Read the model definition and answer for the solid it produces. Units are mm, in the model's axes. Coordinates: 2 decimals unless noted, no trailing zeros. Write each loop counter-clockwise with the first axis right and the second up, starting at its lowest first coordinate (ties: lowest second). Pieces come first, ordered by that corner, then holes. Notation, with made-up numbers: (-16.5, 59.5) -> (25.5, 59.5) arc R16 cw to (25.5, 90.5) -> close; hole circle Ø10 at (-24, 18.25). An arc over 180 degrees is marked (long way). One line per item, written item: value. Start each with the question number.
1. Find section C-C, the plane x = 1. Write down the section's boundary in (y, z).
2. Consider line 1 along X through (y, z) = (-28, 2.05); line 2 along Y through (x, z) = (97.5, 0.7); line 3 along Y through (x, z) = (89.5, 2.3). Determine where each line is inside the solid, lowest interval first.
3. Find section B-B, the plane z = 1.3. State how many separate pieces and enclosed holes the cut face has, and give its area (3 significant figures).
4. Given P1, Ø1.5, axis at y = -108.5, z = 1, coming from the +X side; P2, Ø4, axis at x = 113.5, y = -88, coming from the -Z side; P3, Ø1.5, axis at x = -151.5, z = 1.5, coming from the -Y side; P4, Ø0.9, axis at y = 108.5, z = 1, coming from the -X side, each flat-ended and moving along its own axis, determine where each tip first touches the part or whether it passes through.
5. Find section A-A, the plane y = -16. Write down the section's boundary in (x, z), and give its area (3 significant figures).
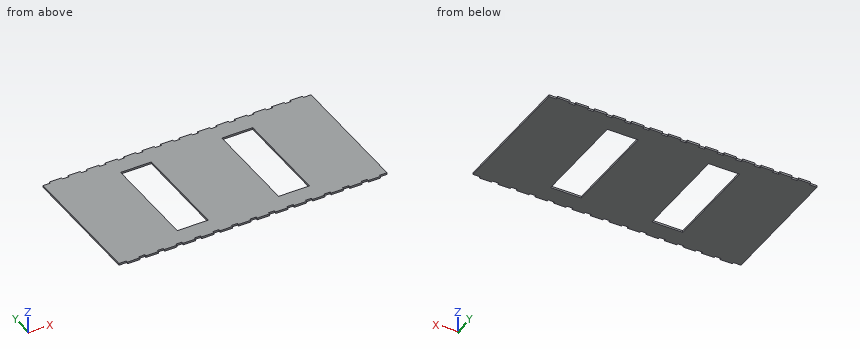
```python
from build123d import *

# Parameters (mm, degrees)
ESQUISSE1_W             = 434
ESQUISSE1_H             = 220
BOSS_EXTRU_1_DEPTH      = 3
ESQUISSE2_W             = 10
ESQUISSE2_H             = 3
ESQUISSE2_W_2           = 2
ENL_V_MAT_EXTRU_1_DEPTH = 3
ESQUISSE3_W             = 50
ESQUISSE3_H             = 160
ENL_V_MAT_EXTRU_2_DEPTH = 3


with BuildPart() as part:
    # Esquisse1 → Boss.-Extru.1 (new body)
    with BuildSketch(Plane.XY):
        Rectangle(ESQUISSE1_W, ESQUISSE1_H)
    extrude(amount=BOSS_EXTRU_1_DEPTH)

    # Esquisse2 → Enlèv. mat.-Extru.1 (cut)
    with BuildSketch(Plane.XY.offset(3)):
        with Locations((-210, 108.5)):
            Rectangle(ESQUISSE2_W, ESQUISSE2_H)
        with Locations((-180, 108.5)):
            Rectangle(ESQUISSE2_W, ESQUISSE2_H)
        with Locations((-150, 108.5)):
            Rectangle(ESQUISSE2_W, ESQUISSE2_H)
        with Locations((-120, 108.5)):
            Rectangle(ESQUISSE2_W, ESQUISSE2_H)
        with Locations((-90, 108.5)):
            Rectangle(ESQUISSE2_W, ESQUISSE2_H)
        with Locations((-30, 108.5)):
            Rectangle(ESQUISSE2_W, ESQUISSE2_H)
        with Locations((30, 108.5)):
            Rectangle(ESQUISSE2_W, ESQUISSE2_H)
        with Locations((60, 108.5)):
            Rectangle(ESQUISSE2_W, ESQUISSE2_H)
        with Locations((90, 108.5)):
            Rectangle(ESQUISSE2_W, ESQUISSE2_H)
        with Locations((120, 108.5)):
            Rectangle(ESQUISSE2_W, ESQUISSE2_H)
        with Locations((150, 108.5)):
            Rectangle(ESQUISSE2_W, ESQUISSE2_H)
        with Locations((180, 108.5)):
            Rectangle(ESQUISSE2_W, ESQUISSE2_H)
        with Locations((210, 108.5)):
            Rectangle(ESQUISSE2_W, ESQUISSE2_H)
        with Locations((210, -108.5)):
            Rectangle(ESQUISSE2_W, ESQUISSE2_H)
        with Locations((180, -108.5)):
            Rectangle(ESQUISSE2_W, ESQUISSE2_H)
        with Locations((150, -108.5)):
            Rectangle(ESQUISSE2_W, ESQUISSE2_H)
        with Locations((90, -108.5)):
            Rectangle(ESQUISSE2_W, ESQUISSE2_H)
        with Locations((60, -108.5)):
            Rectangle(ESQUISSE2_W, ESQUISSE2_H)
        with Locations((-30, -108.5)):
            Rectangle(ESQUISSE2_W, ESQUISSE2_H)
        with Locations((-60, -108.5)):
            Rectangle(ESQUISSE2_W, ESQUISSE2_H)
        with Locations((-90, -108.5)):
            Rectangle(ESQUISSE2_W, ESQUISSE2_H)
        with Locations((-120, -108.5)):
            Rectangle(ESQUISSE2_W, ESQUISSE2_H)
        with Locations((-150, -108.5)):
            Rectangle(ESQUISSE2_W, ESQUISSE2_H)
        with Locations((-210, -108.5)):
            Rectangle(ESQUISSE2_W, ESQUISSE2_H)
        with Locations((-180, -108.5)):
            Rectangle(ESQUISSE2_W, ESQUISSE2_H)
        with Locations((-216, -108.5)):
            Rectangle(ESQUISSE2_W_2, ESQUISSE2_H)
        with Locations((-216, 108.5)):
            Rectangle(ESQUISSE2_W_2, ESQUISSE2_H)
        with Locations((-60, 108.5)):
            Rectangle(ESQUISSE2_W, ESQUISSE2_H)
        with Locations((0, 108.5)):
            Rectangle(ESQUISSE2_W, ESQUISSE2_H)
        with Locations((120, -108.5)):
            Rectangle(ESQUISSE2_W, ESQUISSE2_H)
        with Locations((30, -108.5)):
            Rectangle(ESQUISSE2_W, ESQUISSE2_H)
        with Locations((0, -108.5)):
            Rectangle(ESQUISSE2_W, ESQUISSE2_H)
        with Locations((216, 108.5)):
            Rectangle(ESQUISSE2_W_2, ESQUISSE2_H)
        with Locations((216, -108.5)):
            Rectangle(ESQUISSE2_W_2, ESQUISSE2_H)
    extrude(amount=-ENL_V_MAT_EXTRU_1_DEPTH, mode=Mode.SUBTRACT)

    # Esquisse3 → Enlèv. mat.-Extru.2 (cut)
    with BuildSketch(Plane.XY.offset(3)):
        with Locations((-82, 0)):
            Rectangle(ESQUISSE3_W, ESQUISSE3_H)
        with Locations((82, 0)):
            Rectangle(ESQUISSE3_W, ESQUISSE3_H)
    extrude(amount=-ENL_V_MAT_EXTRU_2_DEPTH, mode=Mode.SUBTRACT)


solid = part.part
```
Answer block:
1. outline: (-107, 0) -> (107, 0) -> (107, 3) -> (-107, 3) -> close
2. line 1: x = -217 to -107, -57 to 57, 107 to 217
2. line 2: y = -110 to -80, 80 to 110
2. line 3: y = -107 to -80, 80 to 107
3. separate pieces: 1
3. enclosed holes: 2
3. area: 78,600 mm2
4. P1: stops at x = 205
4. P2: stops at z = 0
4. P3: stops at y = -107
4. P4: stops at x = -205
5. outline: (-217, 0) -> (-107, 0) -> (-107, 3) -> (-217, 3) -> close; (-57, 0) -> (57, 0) -> (57, 3) -> (-57, 3) -> close; (107, 0) -> (217, 0) -> (217, 3) -> (107, 3) -> close
5. area: 1,000 mm2
